Here's how the part is built. I have some questions about the finished solid (model axes, mm). Face numbers are marked on the shaded views. A direction names the side the tool comes from. Give positions to 0.01 mm unless a question says otherwise; leave off trailing zeros. Loops run counter-clockwise (first coordinate to the right, second up) from the corner with the lowest first, then second, coordinate; pieces in that order, holes last. Notation, with made-up numbers: (-9.5, 7.5) - (20.5, 7.5) arc R36 cw to (20.5, 46.5) - close; hole circle Ø7 at (35.5, -9.75). An arc over 180 degrees is marked (long way). Return JSON: item names as keys, results as strings. Group by question number.
(1) If we section it at D-D (y = 46.5): Please give me the cut outline in (x, z), then the cut area to 3 significant figures.
(2) For P1, Ø4, axis at x = -35, y = 2, coming from the +Z side; P2, Ø3, axis at x = -36.5, z = 9, coming from the -Y side; P3, Ø10, axis at y = 41, z = -22.5, coming from the -X side; P4, Ø5.5, axis at y = 2, z = -35.5, coming from the -X side, each with a flat end and sliding along its axis, tell me the tip position at first contact or that it passes through.
(3) If we mould it in two halves opening along Y, with no side actions, what happens to the marked faces 1, 2 and 3? For each: released by +Y, released by -Y, zero draft, split by the parting line, or undercut.
(4) If we section it at C-C (y = 32.5): Please give me the cut outline in (x, z), then the cut area to 3 significant figures.
(5) I need wall thicknesses on probe 1 along Y at (x, z) = (-26.5, -27); probe 2 along X at (y, z) = (36, -4); probe 3 along Z at (x, y) = (-5, 12). Which ranges of each line are inside material? Lowest first, please. Write a range as [from, to].
(6) On a 3-axis mill with a long thin cutter (end or side, diameter ignored), from which of +Z, -Z, +X, -X, +Y, -Y can I reach the whole of each face in a straight line? I mean the marked faces 4, 5 and 6. Say none if no direction works.
(7) If we section it at B-B (z = 8.5): Please give me the cut outline in (x, y), then the cut area to 3 significant figures.
(8) If we section it at A-A (x = -18): Please give me the cut outline in (y, z), then the cut area to 3 significant figures.
```python
from build123d import *

# Parameters (mm, degrees)
BOSS_EXTRUDE1_DEPTH = 5
BOSS_EXTRUDE2_DEPTH = 58
BOSS_EXTRUDE2_DRAFT = -8


with BuildPart() as part:
    # Sketch1 → Boss-Extrude1 (new body)
    with BuildSketch(Plane(origin=(0, 0, 0), x_dir=(1, 0, 0), z_dir=(0, 1, 0))):
        Polygon((38.97114317, 32.5), (28.867513459, 50), (8.660254038, 50), (-8.660254038, 50), (-28.867513459, 50), (-38.97114317, 32.5), (-47.631397208, 17.5), (-57.735026919, 0), (-47.631397208, -17.5), (-38.97114317, -32.5), (-28.867513459, -50), (-8.660254038, -50), (8.660254038, -50), (28.867513459, -50), (38.97114317, -32.5), (47.631397208, -17.5), (57.735026919, 0), (47.631397208, 17.5), align=None)
        Polygon((-20, -40.414518843), (-25, -37.527767497), (-25, -31.754264805), (-20, -28.867513459), (-15, -31.754264805), (-15, -37.527767497), align=None, mode=Mode.SUBTRACT)
        Polygon((2.886751346, -45), (-2.886751346, -45), (-5.773502692, -40), (-2.886751346, -35), (2.886751346, -35), (5.773502692, -40), align=None, mode=Mode.SUBTRACT)
        Polygon((-37.527767497, -25), (-40.414518843, -20), (-37.527767497, -15), (-31.754264805, -15), (-28.867513459, -20), (-31.754264805, -25), align=None, mode=Mode.SUBTRACT)
        Polygon((-2.886751346, -25), (-5.773502692, -20), (-2.886751346, -15), (2.886751346, -15), (5.773502692, -20), (2.886751346, -25), align=None, mode=Mode.SUBTRACT)
        Polygon((-23.094010768, -10), (-20.207259422, -5), (-14.43375673, -5), (-11.547005384, -10), (-14.43375673, -15), (-20.207259422, -15), align=None, mode=Mode.SUBTRACT)
        Polygon((25, -37.527767497), (20, -40.414518843), (15, -37.527767497), (15, -31.754264805), (20, -28.867513459), (25, -31.754264805), align=None, mode=Mode.SUBTRACT)
        Polygon((40.414518843, -20), (37.527767497, -25), (31.754264805, -25), (28.867513459, -20), (31.754264805, -15), (37.527767497, -15), align=None, mode=Mode.SUBTRACT)
        Polygon((20.207259422, -15), (14.43375673, -15), (11.547005384, -10), (14.43375673, -5), (20.207259422, -5), (23.094010768, -10), align=None, mode=Mode.SUBTRACT)
        Polygon((45, 2.886751346), (45, -2.886751346), (40, -5.773502692), (35, -2.886751346), (35, 2.886751346), (40, 5.773502692), align=None, mode=Mode.SUBTRACT)
        Polygon((-45, -2.886751346), (-45, 2.886751346), (-40, 5.773502692), (-35, 2.886751346), (-35, -2.886751346), (-40, -5.773502692), align=None, mode=Mode.SUBTRACT)
        Polygon((-20.207259422, 15), (-14.43375673, 15), (-11.547005384, 10), (-14.43375673, 5), (-20.207259422, 5), (-23.094010768, 10), align=None, mode=Mode.SUBTRACT)
        Polygon((-40.414518843, 20), (-37.527767497, 25), (-31.754264805, 25), (-28.867513459, 20), (-31.754264805, 15), (-37.527767497, 15), align=None, mode=Mode.SUBTRACT)
        Polygon((-25, 37.527767497), (-20, 40.414518843), (-15, 37.527767497), (-15, 31.754264805), (-20, 28.867513459), (-25, 31.754264805), align=None, mode=Mode.SUBTRACT)
        Polygon((23.094010768, 10), (20.207259422, 5), (14.43375673, 5), (11.547005384, 10), (14.43375673, 15), (20.207259422, 15), align=None, mode=Mode.SUBTRACT)
        Polygon((37.527767497, 25), (40.414518843, 20), (37.527767497, 15), (31.754264805, 15), (28.867513459, 20), (31.754264805, 25), align=None, mode=Mode.SUBTRACT)
        Polygon((2.886751346, 25), (5.773502692, 20), (2.886751346, 15), (-2.886751346, 15), (-5.773502692, 20), (-2.886751346, 25), align=None, mode=Mode.SUBTRACT)
        Polygon((20, 40.414518843), (25, 37.527767497), (25, 31.754264805), (20, 28.867513459), (15, 31.754264805), (15, 37.527767497), align=None, mode=Mode.SUBTRACT)
        Polygon((-2.886751346, 45), (2.886751346, 45), (5.773502692, 40), (2.886751346, 35), (-2.886751346, 35), (-5.773502692, 40), align=None, mode=Mode.SUBTRACT)
    extrude(amount=BOSS_EXTRUDE1_DEPTH)


with BuildPart() as boss_extrude2_tool:
    # Sketch2 → Boss-Extrude2 (with draft: the straight prism first)
    with BuildSketch(Plane(origin=(0, 0, 0), x_dir=(1, 0, 0), z_dir=(0, 1, 0))):
        Polygon((7.505553499, -13), (15.011106999, 0), (7.505553499, 13), (-7.505553499, 13), (-15.011106999, 0), (-7.505553499, -13), align=None)
    extrude(amount=BOSS_EXTRUDE2_DEPTH)
    # Boss-Extrude2: the draft: its side faces are tilted about the plane it starts from
    boss_extrude2_sides = [boss_extrude2_tool.faces().sort_by_distance(p)[0] for p in [
        (11.258330249, 29, 6.5),
        (11.258330249, 29, -6.5),
        (0, 29, -13),
        (-11.258330249, 29, -6.5),
        (-11.258330249, 29, 6.5),
        (0, 29, 13),
    ]]
    draft(boss_extrude2_sides, Plane(origin=(0, 0, 0), x_dir=(1, 0, 0), z_dir=(0, 1, 0)), BOSS_EXTRUDE2_DRAFT)


with BuildPart() as part_1:
    add(part.part)

    # Boss-Extrude2: add boss_extrude2_tool
    add(boss_extrude2_tool.part)


solid = part_1.part
```
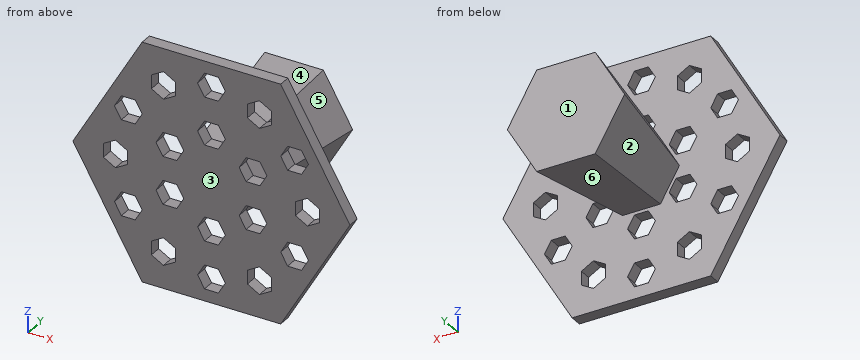
Values:
{
 "1": {"outline": "(-22.56, 0) - (-11.28, -19.54) - (11.28, -19.54) - (22.56, 0) - (11.28, 19.54) - (-11.28, 19.54) - close", "area": "1,320 mm2"},
 "2": {"P1": "z = 42.84", "P2": "y = 0", "P3": "x = -11.67", "P4": "x = -38.83"},
 "3": {"face 1": "released by +Y", "face 2": "undercut", "face 3": "released by -Y"},
 "4": {"outline": "(-20.29, 0) - (-10.14, -17.57) - (10.14, -17.57) - (20.29, 0) - (10.14, 17.57) - (-10.14, 17.57) - close", "area": "1,070 mm2"},
 "5": {"probe 1": "[0, 5]", "probe 2": "[-18.54, 18.54]", "probe 3": "[-14.69, 14.69]"},
 "6": {"face 4": "+Z, +X, -X", "face 5": "+Z, +X", "face 6": "-Z, +X, -X"},
 "7": {"outline": "(-52.83, 0) - (-22.23, 0) - (-22.23, 5) - (-52.83, 5) - close; (-19.52, 58) - (-10.92, 5) - (-12.41, 5) - (-12.41, 0) - (12.41, 0) - (12.41, 5) - (10.92, 5) - (19.52, 58) - close; (22.23, 0) - (52.83, 0) - (52.83, 5) - (22.23, 5) - close", "area": "2,040 mm2"},
 "8": {"outline": "(0, -50) - (5, -50) - (5, -39.26) - (0, -39.26) - close; (0, -30.02) - (5, -30.02) - (5, -15) - (0, -15) - close; (0, -5) - (5, -5) - (5, 5) - (0, 5) - close; (0, 15) - (5, 15) - (5, 30.02) - (0, 30.02) - close; (0, 39.26) - (5, 39.26) - (5, 50) - (0, 50) - close; (18.42, 0) - (58, -11.13) - (58, 11.13) - close", "area": "748 mm2"}
}
